Could you check a few things on this model? Use its own coordinates, in mm. A direction names the side the tool comes from. Coordinates: 2 decimals unless noted, no trailing zeros. Write each loop counter-clockwise with the first axis right and the second up, starting at its lowest first coordinate (ties: lowest second). Pieces come first, ordered by that corner, then holes. Notation, with made-up numbers: M 81,63 L 109,63 A11 cw 109,71 Z; hole C 8,85.5 d10. An arc over 180 degrees is marked long. Answer as CSV lines item,"result". Start each with the question number.
Item 1: If I drill on line 1 along Z through (x, y) = (-3, 54); line 2 along X through (y, z) = (3, 30); line 3 along Y through (x, z) = (-15, 27), over which ranges is the centre line in solid material (lowest first)? Write a range as [from, to].
Item 2: Suppose I cut it at A-A, the plane z = 30. State how many separate pieces and enclosed holes the cut face has, and give its area (3 significant figures).
Item 3: I'm going to push flat-ended pins straight in: P1, Ø7, axis at y = 54, z = 30, coming from the +X side; P2, Ø7.5, axis at y = 72, z = 16, coming from the -X side; P3, Ø7, axis at x = -21.5, z = 2.5, coming from the +Y side; P4, Ø10.5, axis at x = -73, z = -13.5, coming from the +Y side. Where does each tip first touch, or does it pass through?
Item 4: Suppose I cut it at B-B, the plane y = 51. Write out the boundary of the cut face in (x, z), and give its area (3 significant figures).
Item 5: Suppose I cut it at C-C, the plane y = 70. Write out the boundary of the cut face in (x, z).
Item 6: On a 3-axis mill with a long thin cutter (end or side, diameter ignored), from which of +Z, -Z, +X, -X, +Y, -Y can I reach the whole of each face in a straight line? I mean faces 5 (the cylindrical face through (-55.96, 4.06, 26.23)), 6 (the flat face through (-8, 35, 1)), 7 (the cylindrical face through (-14.9, 9.1, 0.7)). Say none if no direction works.
Item 7: We'd pull the mould along X, two halves only. Please class faces 1 (the flat face through (-8, 61, 1)), 2 (the cylindrical face through (-55.96, 4.06, -33.77)), 3 (the flat face through (-47, 8, 1)), 4 (the flat face through (-16.38, 16.67, 0.69)): +X half, -X half, draft (parallel to the pull), parting line (faces both ways), or undercut.
```python
from build123d import *

# Parameters (mm, degrees)
EXTRUDE_1_DEPTH     = 49
SKETCH_2_R          = 4.25
CUT_EXTRUDE_1_DEPTH = 9
SKETCH_3_R          = 4.25
CUT_EXTRUDE_2_DEPTH = 9


with BuildPart() as part:
    # Эскиз1 → Бобышка-Вытянуть1 (new body, symmetric)
    with BuildSketch(Plane.XY):
        Polygon((-78, 0), (0, 0), (0, 78), (-8, 78), (-8, 68.5), (-7.5, 68), (-8, 67.5), (-8, 54.5), (-7.5, 54), (-8, 53.5), (-8, 40.5), (-7.5, 40), (-8, 39.5), (-8, 30), (-30, 8), (-39.5, 8), (-40, 7.5), (-40.5, 8), (-53.5, 8), (-54, 7.5), (-54.5, 8), (-67.5, 8), (-68, 7.5), (-68.5, 8), (-78, 8), align=None)
        with BuildLine():
            Line((-4.5, 12), (-4.5, 26.136038969))
            ThreePointArc((-4.5, 26.136038969), (-5.117316568, 27.059918502), (-6.207106781, 26.843145751))
            Line((-6.207106781, 26.843145751), (-26.843145751, 6.207106781))
            ThreePointArc((-26.843145751, 6.207106781), (-27.059918502, 5.117316568), (-26.136038969, 4.5))
            Line((-26.136038969, 4.5), (-12, 4.5))
            Line((-12, 4.5), (-12, 7.9))
            ThreePointArc((-12, 7.9), (-14.899137803, 9.100862197), (-16.1, 12))
            ThreePointArc((-16.1, 12), (-15.1, 13), (-14.1, 12))
            ThreePointArc((-14.1, 12), (-10.51507576, 10.51507576), (-12, 14.1))
            ThreePointArc((-12, 14.1), (-13, 15.1), (-12, 16.1))
            ThreePointArc((-12, 16.1), (-9.100862197, 14.899137803), (-7.9, 12))
            Line((-7.9, 12), (-4.5, 12))
        make_face(mode=Mode.SUBTRACT)
    extrude(amount=EXTRUDE_1_DEPTH, both=True)

    # Эскиз2 → Вырез-Вытянуть1 (cut, through all)
    with BuildSketch(Plane.ZY.offset(8)):
        with Locations(Location((-30, 54, 0), (0, 0, 270))):  # turned: the seam where the file's is
            Circle(SKETCH_2_R)
        with Locations(Location((30, 54, 0), (0, 0, 270))):  # turned: the seam where the file's is
            Circle(SKETCH_2_R)
    extrude(amount=-CUT_EXTRUDE_1_DEPTH, mode=Mode.SUBTRACT)

    # Эскиз3 → Вырез-Вытянуть2 (cut, through all)
    with BuildSketch(Plane(origin=(0, 8, 0), x_dir=(1, 0, 0), z_dir=(0, 1, 0))):
        with Locations(Location((-54, -30, 0), (0, 0, 180))):  # turned: the seam where the file's is
            Circle(SKETCH_3_R)
        with Locations(Location((-54, 30, 0), (0, 0, 180))):  # turned: the seam where the file's is
            Circle(SKETCH_3_R)
    extrude(amount=-CUT_EXTRUDE_2_DEPTH, mode=Mode.SUBTRACT)


solid = part.part
```
Ans:
1,line 1,"z = [-49, -34.25], [-25.75, 25.75], [34.25, 49]"
1,line 2,"x = [-78, -58.25], [-49.75, 0]"
1,line 3,"y = [0, 4.5], [9.21, 12.99], [18.05, 23]"
2,separate pieces,"3"
2,enclosed holes,"1"
2,area,"1,080 mm^2"
3,P1,"passes through"
3,P2,"stops at x = -8"
3,P3,"stops at y = 20"
3,P4,"stops at y = 8"
4,outline,"M -8,-49 L 0,-49 L 0,-33.01 L -8,-33.01 Z; M -8,-26.99 L 0,-26.99 L 0,26.99 L -8,26.99 Z; M -8,33.01 L 0,33.01 L 0,49 L -8,49 Z"
4,area,"688 mm^2"
5,outline,"M -8,-49 L 0,-49 L 0,49 L -8,49 Z"
6,face 5,"+Y, -Y"
6,face 6,"+Z, -Z, -X, +Y"
6,face 7,"+Z, -Z"
7,face 1,"-X half"
7,face 2,"undercut"
7,face 3,"draft"
7,face 4,"undercut"
